The listing builds one solid part. Answer for the finished solid, in the listing's coordinates (mm). Coordinates: 2 decimals unless noted, no trailing zeros. Order: outer loops, then holes, each group sorted by start corner. A loop starts at its lowest first (then second) coordinate and runs counter-clockwise, first axis right, second up. Notation, with made-up numbers: (-22.75, 51) -> (22.25, 51) arc R14 cw to (22.25, 74) -> close; hole circle Ø2 at (-33.75, 49.5). An arc over 180 degrees is marked (long way). Return JSON: item names as keys, results as strings.
Autodesk Fusion 360 part; units mm, degrees
sketch "Sketch1" plane through (0, 0, 0) normal (0, 0, 1) x (1, 0, 0)
  line L0 (167.6875, -186.5) -> (-20, -186.5)
  line L1 (-10, 15) -> (157.6875, 15)
  line L2 (-20, -186.5) -> (-20, 25)
  line L3 (167.6875, 25) -> (167.6875, -186.5)
  line L4 (-10, -176.5) -> (-10, 15)
  line L5 (157.6875, 15) -> (157.6875, -176.5)
  line L6 (157.6875, -176.5) -> (-10, -176.5)
  line L7 (-20, 25) -> (167.6875, 25)
  line L8 (15, -176.5) -> (-5, -176.5)
  line L9 (-5, -176.5) -> (-5, -186.5)
  line L10 (-5, -186.5) -> (15, -186.5)
  line L11 (15, -186.5) -> (15, -176.5)
  line L12 (-10, 15) -> (18, 15)
  line L13 (18, 15) -> (18, -141)
  line L14 (18, -141) -> (-10, -141)
  line L15 (-10, -141) -> (-10, 15)
  line L16 (44, 15) -> (54, 15)
  line L17 (54, 15) -> (54, -141)
  line L18 (54, -141) -> (44, -141)
  line L19 (44, -141) -> (44, 15)
  line L20 (157.6875, -176.5) -> (121.6875, -176.5)
  line L21 (121.6875, -176.5) -> (121.6875, -141)
  line L22 (121.6875, -141) -> (157.6875, -141)
  line L23 (157.6875, -141) -> (157.6875, -176.5)
  line L24 (44, -141) -> (121.6875, -141)
  line L25 (121.6875, -141) -> (121.6875, -151)
  line L26 (121.6875, -151) -> (44, -151)
  line L27 (44, -151) -> (44, -141)
  line L28 (44, -151) -> (18, -151)
  line L29 (18, -151) -> (18, -141)
  line L30 (18, -141) -> (44, -141)
  line L31 (44, -141) -> (44, -151)
  line L32 (14, -141) -> (18, -141)
  line L33 (18, -141) -> (18, -151)
  line L34 (18, -151) -> (14, -151)
  line L35 (14, -151) -> (14, -141)
  dimension "d3" = 167.6875
  dimension "d4" = 191.5
  dimension "d5" = 187.6875
  dimension "d6" = 211.5
  dimension "d7" = 10
  dimension "d8" = 10
  dimension "d19" = 20
  dimension "d20" = 15
  dimension "d21" = 28
  dimension "d22" = 156
  dimension "d23" = 10
  dimension "d24" = 156
  dimension "d25" = 26
  dimension "d26" = 36
  dimension "d27" = 35.5
  dimension "d28" = 10
extrude "Extrude1" add sketch "Sketch1" along normal blind 2 contours L0 L1 L2 L3 L4 L5 L6 L7 L9 L11 L12 L15 L16 L20 L23 | L5 L6 L20 L21 L22 L23 L25 | L18 L21 L24 L25 L26 L27 L31 | L1 L4 L12 L13 L14 L15 L32 | L27 L28 L29 L30 L31 L33 | L14 L29 L32 L33 L34 L35 | L1 L16 L17 L18 L19 L24
fillet "Fillet1" radius 6 1 edges at (167.6875, -186.5, 1)
fillet "Fillet2" radius 6 1 edges at (167.6875, 25, 1)
fillet "Fillet3" radius 6 1 edges at (-20, 25, 1)
fillet "Fillet4" radius 6 1 edges at (-20, -186.5, 1)
sketch "Sketch2" plane through (0, 0, 2) normal (0, 0, 1) x (-1, 0, 0)
  arc A0 (20, 180.5) -> (14, 186.5) centre (14, 180.5) ccw
  line L0 (14, 186.5) -> (5, 186.5)
  line L1 (5, 186.5) -> (5, 176.5)
  line L2 (5, 176.5) -> (10, 176.5)
  line L3 (10, 176.5) -> (10, 141)
  line L4 (10, 141) -> (-14, 141)
  line L5 (-14, 141) -> (-14, 151)
  line L6 (-14, 151) -> (-121.6875, 151)
  line L7 (-121.6875, 151) -> (-121.6875, 176.5)
  line L8 (-121.6875, 176.5) -> (-15, 176.5)
  line L9 (-15, 176.5) -> (-15, 186.5)
  line L10 (-15, 186.5) -> (-161.6875, 186.5)
  arc A1 (-161.6875, 186.5) -> (-167.6875, 180.5) centre (-161.6875, 180.5) ccw
  line L11 (-167.6875, 180.5) -> (-167.6875, -19)
  arc A2 (-167.6875, -19) -> (-161.6875, -25) centre (-161.6875, -19) ccw
  line L12 (-161.6875, -25) -> (14, -25)
  arc A3 (14, -25) -> (20, -19) centre (14, -19) ccw
  line L13 (20, -19) -> (20, 180.5)
  line L14 (-18, 141) -> (-18, -15)
  line L15 (-18, -15) -> (-44, -15)
  line L16 (-44, -15) -> (-44, 141)
  line L17 (-44, 141) -> (-18, 141)
  line L18 (-54, -15) -> (-157.6875, -15)
  line L19 (-157.6875, -15) -> (-157.6875, 141)
  line L20 (-157.6875, 141) -> (-54, 141)
  line L21 (-54, 141) -> (-54, -15)
  circle A4 centre (14, -19) radius 2.1
  circle A5 centre (-161.6875, -19) radius 2.1
  circle A6 centre (-161.6875, 180.5) radius 2.1
  circle A7 centre (14, 180.5) radius 2.1
  dimension "d29" = 4.2
  dimension "d30" = 4.2
  dimension "d31" = 4.2
  dimension "d32" = 4.2
  dimension "d33" = 6
  dimension "d34" = 6
  dimension "d35" = 6
  dimension "d36" = 6
  dimension "d37" = 6
  dimension "d38" = 6
  dimension "d39" = 6
  dimension "d40" = 6
extrude "Extrude2" add sketch "Sketch2" against normal blind 6 contours A4 | A5 | A6 | A7
1. Each of these flat-tipped pins is pushed along its axis until it touches: pin 1 Ø1.6 at (x, z) = (-1, 1) entering from -Y; pin 2 Ø2 at (y, z) = (-63.5, -2.5) entering from -X; pin 3 Ø1 at (y, z) = (-183.5, 0.5) entering from -X. Where does it stop, or does it pass through?
Answer block:
{"pin 1": "stops at y = -141", "pin 2": "passes through", "pin 3": "stops at x = -19.45"}
2. The part is cut by section A-A on y = -54. Give the vertices of the cut face in (x, z).
Answer block:
{"outline": "(-20, 0) -> (18, 0) -> (18, 2) -> (-20, 2) -> close; (44, 0) -> (54, 0) -> (54, 2) -> (44, 2) -> close; (157.69, 0) -> (167.69, 0) -> (167.69, 2) -> (157.69, 2) -> close"}
3. The part is cut by section B-B on z = -1.15. Give the vertices of the cut face in (x, y).
Answer block:
{"outline": "circle Ø4.2 at (-14, -180.5); circle Ø4.2 at (-14, 19); circle Ø4.2 at (161.69, -180.5); circle Ø4.2 at (161.69, 19)"}
4. Determine the mould class of faces 1 (the face through (-18.196, 23.289, 1.014)), 2 (the face through (165.88, -184.79, 1.01)), 3 (the face through (52, -79, 2)) for opening direction Y: pulls with the +Y half, pulls with the -Y half, needs draft (parallel to the pull), parting line crosses it, or undercut.
Answer block:
{"face 1": "pulls with the +Y half", "face 2": "pulls with the -Y half", "face 3": "needs draft"}
5. Consider line 1 (X direction, y = -26.5, z = 1.15); line 2 (Y direction, x = 112, z = 0.9); line 3 (Y direction, x = 141.5, z = 1.75). Determine where each line is inside the solid, lowest interval first. Write a range as from..to.
Answer block:
{"line 1": "x = -20..18, 44..54, 157.69..167.69", "line 2": "y = -186.5..-176.5, -151..-141, 15..25", "line 3": "y = -186.5..-141, 15..25"}
